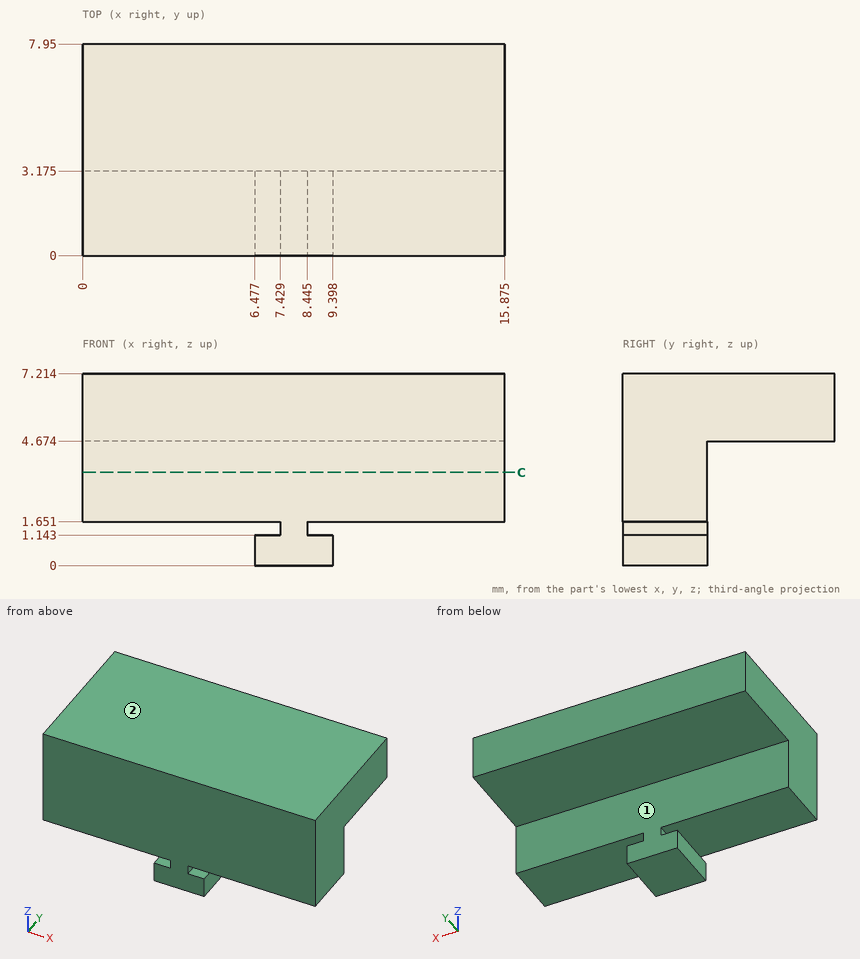
Print and shaded views of the part. All mm, measured from the part's lowest x, y and z. A direction names the side the tool comes from. Give positions to 0.01 mm unless a question says otherwise; leave off trailing zeros. Order: outer loops, then holes, each group sorted by start corner. A loop starts at its lowest first (then second) coordinate and runs counter-clockwise, first axis right, second up. Notation, with made-up numbers: (84, 21.25) - (128, 21.25) arc R35 cw to (128, 54.25) - close; hole circle Ø4 at (78, 17.5). An arc over 180 degrees is marked (long way). One line per item, written item: value.
Item 1: Tool access for the marked faces 1 and 2: list every direction of +Z, -Z, +X, -X, +Y, -Y with a clear straight run to the whole face (end or side of a thin tool).
Response values:
face 1: -Z, +X, -X, +Y
face 2: +Z, +X, -X, +Y, -Y
Item 2: Pin check, flat tips, straight feed: pin 1 Ø1 at (x, z) = (12.5, 1.5) entering from +Y (1 decimal); pin 2 Ø4 at (x, y) = (9.5, 6) entering from -Z; pin 3 Ø1.5 at (y, z) = (5.5, 2) entering from -X; pin 4 Ø2.5 at (x, y) = (2.5, 1.5) entering from -Z. Stop position of each tip, or through.
Response values:
pin 1: y = 3.2
pin 2: z = 4.67
pin 3: through
pin 4: z = 1.65
Item 3: Wall check: line 1 (Y direction, x = 15, z = 3.5) (1 decimal); line 2 (Z direction, x = 8.5, y = 4); line 3 (Z direction, x = 12.5, y = 0.5). Give the ranges that are in metal, low to high.
Response values:
line 1: 0 to 3.2
line 2: 4.67 to 7.21
line 3: 1.65 to 7.21
Item 4: Slice it at C-C (z = 3.5). List the corners of the cut face in (x, y) (1 decimal).
Response values:
outline: (0, 0) - (15.9, 0) - (15.9, 3.2) - (0, 3.2) - close
